Can you work these out from the model? Positions are in its coordinate system, mm. A direction names the side the tool comes from. Give positions to 0.01 mm unless a question says otherwise; leave off trailing zeros. Write each loop counter-clockwise with the first axis right and the second up, starting at its lowest first coordinate (ties: lowest second). Pieces come first, ordered by that corner, then holes.
1. If I drill on probe 1 along Z at (x, y) = (-1.5, 0); probe 2 along Y at (x, z) = (-5.25, 1.5); probe 3 along Z at (x, y) = (-6.5, 10), over which ranges is the centre line in solid material (lowest first)?
2. Suppose I cut it at D-D (z = 17). Please give me the cut outline in (x, y).
3. On a 3-axis mill with a long thin cutter (end or side, diameter ignored), from which of +Z, -Z, +X, -X, +Y, -Y can I reach the whole of each face in a straight line? I mean faces 1 (the cylindrical face through (-8.99, 12.85, 20.15)), 2 (the cylindrical face through (-5.056, 9.443, -2.974)), 3 (the flat face through (0, 2, -22)). Say none if no direction works.
4. Suppose I cut it at C-C (x = -5.75). Please give me the cut outline in (y, z), and give its area (3 significant figures).
5. I'm going to push flat-ended pins straight in: pin 1 (5 mm diameter, centred on x = -2.5, y = -7.5, fed in from +Z); pin 2 (6 mm diameter, centred on x = -3, y = 4, fed in from +Z); pin 3 (13 mm diameter, centred on y = -4, z = -1.5, fed in from +X). Where does each tip first touch, or does it pass through?
6. Thinking about a two-plate mould opening in Y: for faces 4 (the cylindrical face through (-3.94, -18.35, 16.83)), 5 (the flat face through (-8, -9.3, 22.2)), 6 (the cylindrical face through (-9.51, -1.93, 8.69)), which applies, pulls with the +Y half, pulls with the -Y half, needs draft (parallel to the pull), parting line crosses it, or undercut?
7. Suppose I cut it at A-A (y = 0). Please give me the cut outline in (x, z), and give its area (3 significant figures).
Autodesk Inventor part; units mm, degrees
ref_plane "YZ Plane" through (0, 0, 0) normal (1, 0, 0) x (0, 1, 0)
ref_plane "XZ Plane" through (0, 0, 0) normal (0, 1, 0) x (-1, 0, 0)
ref_plane "XY Plane" through (0, 0, 0) normal (0, 0, 1) x (1, 0, 0)
sketch "Sketch1" plane through (0, 0, 0) normal (0, 0, 1) x (1, 0, 0)
  line L0 (-12, 0) -> (2, 0) construction
  line L1 (0, -4.98) -> (0, 29.88) construction
  line L2 (0, 9.9) -> (-9, 9.9)
  line L3 (-9, 9.9) -> (-9, 8.9)
  line L4 (-9, 8.9) -> (-10, 8.9)
  line L5 (-10, 8.9) -> (-10, 23.9)
  line L6 (-10, 23.9) -> (-8, 23.9)
  line L7 (-8, 23.9) -> (-8, 24.9)
  line L8 (-8, 24.9) -> (0, 24.9)
  line L9 (0, 21.9) -> (-7, 21.9)
  line L10 (-7, 21.9) -> (-7, 12.9)
  line L11 (-7, 12.9) -> (0, 12.9)
  line L12 (0, 24.9) -> (0, 21.9)
  line L13 (0, 12.9) -> (0, 9.9)
  point P0 (0, 0)
  dimension "d0" = 49.8
  dimension "d1" = 47.8
  dimension "d3" = 1
  dimension "d4" = 2
  dimension "d5" = 19.8
  dimension "d6" = 1
  dimension "d7" = 3
  dimension "d8" = 3
  dimension "d9" = 3
  dimension "d10" = 10
revolve "Revolution1" add sketch "Sketch1" angle 360 about axis through (-10, 0, 0) along (1, 0, 0)
chamfer "Chamfer1" distance 1 angle 45 1 edges at (0, -9.9, 0)
properties part number "P114PorteLentille20mm" material "ABS Plastic"
Checks:
1. probe 1: z = -24.9 to -21.9, -12.9 to -9.9, 9.9 to 12.9, 21.9 to 24.9
1. probe 2: y = -24.85 to -21.85, -12.81 to -9.79, 9.79 to 12.81, 21.85 to 24.85
1. probe 3: z = -22.8 to -19.48, -8.15 to 8.15, 19.48 to 22.8
2. outline: (-10, -16.8) - (-8, -16.8) - (-8, -18.19) - (0, -18.19) - (0, -13.81) - (-7, -13.81) - (-7, 13.81) - (0, 13.81) - (0, 18.19) - (-8, 18.19) - (-8, 16.8) - (-10, 16.8) - close
3. face 1: -X
3. face 2: +X
3. face 3: +Z, -Z, +X, +Y, -Y
4. outline: circle Ø49.8 at (0, 0); circle Ø25.8 at (0, 0); hole circle Ø43.8 at (0, 0); hole circle Ø19.8 at (0, 0)
4. area: 656 mm2
5. pin 1: stops at z = 24.39
5. pin 2: stops at z = 24.88
5. pin 3: stops at x = -0.13
6. face 4: parting line crosses it
6. face 5: needs draft
6. face 6: undercut
7. outline: (-10, -23.9) - (-8, -23.9) - (-8, -24.9) - (0, -24.9) - (0, -21.9) - (-7, -21.9) - (-7, -12.9) - (0, -12.9) - (0, -10.9) - (-1, -9.9) - (-9, -9.9) - (-9, -8.9) - (-10, -8.9) - close; (-10, 8.9) - (-9, 8.9) - (-9, 9.9) - (-1, 9.9) - (0, 10.9) - (0, 12.9) - (-7, 12.9) - (-7, 21.9) - (0, 21.9) - (0, 24.9) - (-8, 24.9) - (-8, 23.9) - (-10, 23.9) - close
7. area: 171 mm2
